Can you work these out from the model? Positions are in its coordinate system, mm. Give positions to 0.01 mm unless a question says otherwise; leave off trailing zeros. Order: outer loops, then holes, each group sorted by start corner. A loop starts at its lowest first (then second) coordinate and runs counter-clockwise, first axis right, second up. Notation, with made-up numbers: (-20.5, 60) -> (16.5, 60) arc R17 ccw to (16.5, 92) -> close; hole circle Ø10 at (60, -33.75). An arc over 180 degrees is marked (long way). Answer as CSV lines item,"result".
```python
from build123d import *

# Parameters (mm, degrees)
BOSS_EXTRUDE1_DEPTH      = 222.25
BOSS_EXTRUDE1_DEPTH_BACK = 222.25
SKETCH2_W                = 50.8
SKETCH2_H                = 25.4
SKETCH2_W_2              = 47.625
SKETCH2_H_2              = 22.225
SKETCH4_R                = 2.4892
CUT_EXTRUDE2_DEPTH       = 352.780830205


with BuildPart() as part:
    # Sketch2 → Boss-Extrude1 (new, two sides: drawn at the far end of the back side and taken through both)
    with BuildSketch(Plane(origin=(0, 0, 0), x_dir=(0, 0, -1), z_dir=(1, 0, 0)).offset(-BOSS_EXTRUDE1_DEPTH_BACK)):
        with Locations((215.9, 114.3)):
            Rectangle(SKETCH2_W, SKETCH2_H)
        with Locations((215.9, 114.3)):
            Rectangle(SKETCH2_W_2, SKETCH2_H_2, mode=Mode.SUBTRACT)
    extrude(amount=BOSS_EXTRUDE1_DEPTH + BOSS_EXTRUDE1_DEPTH_BACK)

    # Sketch4 → Cut-Extrude2 (cut, through all)
    with BuildSketch(Plane(origin=(0, 0, 0), x_dir=(1, 0, 0), z_dir=(0, 1, 0))):
        with Locations(Location((150.8125, 215.9, 0), (0, 0, 270))):
            Circle(SKETCH4_R)
        with Locations(Location((188.9125, 215.9, 0), (0, 0, 270))):
            Circle(SKETCH4_R)
    cut_extrude2 = extrude(amount=CUT_EXTRUDE2_DEPTH, mode=Mode.SUBTRACT)

    # Mirror2: Cut-Extrude2 across plane
    add(cut_extrude2.mirror(Plane(origin=(0, 0, 0), x_dir=(0, 0, 1), z_dir=(1, 0, 0))), mode=Mode.SUBTRACT)


solid = part.part
```
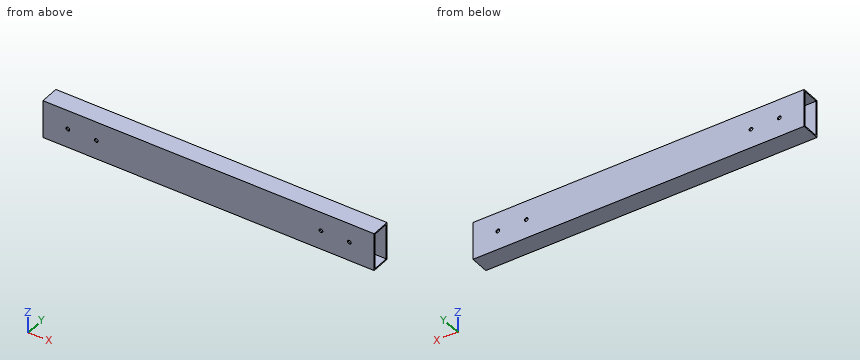
Item 1: Please list where these lines run through material, in increasing order: line 1 along X through (y, z) = (102.7, -215.9); line 2 along Y through (x, z) = (117.5, -194.5); line 3 along Z through (x, y) = (12.5, 113).
Numbers:
line 1,"x = -222.25 to -191.4, -186.42 to -153.3, -148.32 to 148.32, 153.3 to 186.42, 191.4 to 222.25"
line 2,"y = 101.6 to 103.19, 125.41 to 127"
line 3,"z = -241.3 to -239.71, -192.09 to -190.5"
Item 2: Imagine slicing it at B-B, the plane y = 117. Please give me the cut outline in (x, z).
Numbers:
outline,"(-222.25, -241.3) -> (222.25, -241.3) -> (222.25, -239.71) -> (-222.25, -239.71) -> close; (-222.25, -192.09) -> (222.25, -192.09) -> (222.25, -190.5) -> (-222.25, -190.5) -> close"
Item 3: Imagine slicing it at A-A, the plane z = -206. Please give me the cut outline in (x, y), then the cut area to 3 significant figures.
Numbers:
outline,"(-222.25, 101.6) -> (222.25, 101.6) -> (222.25, 103.19) -> (-222.25, 103.19) -> close; (-222.25, 125.41) -> (222.25, 125.41) -> (222.25, 127) -> (-222.25, 127) -> close"
area,"1,410 mm²"
Item 4: Imagine slicing it at C-C, the plane x = -2. Please give me the cut outline in (y, z), then the cut area to 3 significant figures.
Numbers:
outline,"(101.6, -241.3) -> (127, -241.3) -> (127, -190.5) -> (101.6, -190.5) -> close; hole (103.19, -239.71) -> (125.41, -239.71) -> (125.41, -192.09) -> (103.19, -192.09) -> close"
area,"232 mm²"
